from build123d import *

# Parameters (mm, degrees)
F_5_16_CLEARANCE_HOLE1_D = 8.4328
CIRPATTERN1_COUNT        = 8
F_1_2_CLEARANCE_HOLE1_D  = 13.49248
CIRPATTERN2_COUNT        = 2


with BuildPart() as part:
    # Sketch1 → Revolve1 (revolve)
    with BuildSketch(Plane.XY):
        Polygon((-19.431, 0), (-50.8, 0), (-50.8, 12.7), (-19.05, 12.7), (-19.05, 25.4), (0, 25.4), (0, 0), (-15.875, 0), (-15.875, 2.54), (-19.431, 2.54), align=None)
    revolve(axis=Axis((0, 25.4, 0), (0, -1, 0)))

    # Sketch4 → 1/2 NPT Tapped Hole1 (revolve, cut)
    with BuildSketch(Plane(origin=(0, 25.4, 0), x_dir=(0, 0, 1), z_dir=(1, 0, 0))):
        Polygon((0, 0), (0, 25.4), (8.9281, 25.4), (8.9281, 13.462), (9.479726792, 13.462), (9.8827971, 0), align=None)
    revolve(axis=Axis((0, 31.75, 0), (0, -1, 0)), mode=Mode.SUBTRACT)

    # 5/16 Clearance Hole1 (through all)
    with Locations(Plane(origin=(0, 12.7, 0), x_dir=(1, 0, 0), z_dir=(0, 1, 0))):
        with Locations((44.45, 0)):
            f_5_16_clearance_hole1 = Hole(F_5_16_CLEARANCE_HOLE1_D / 2)

    # CirPattern1: 5/16 Clearance Hole1 ×8 about axis
    cirpattern1_axis = Axis((0, 0, 0), (0, 1, 0))
    for i in range(1, CIRPATTERN1_COUNT):
        add(f_5_16_clearance_hole1.rotate(cirpattern1_axis, i * 360 / CIRPATTERN1_COUNT), mode=Mode.SUBTRACT)

    # 1/2 Clearance Hole1 (through all)
    with Locations(Plane(origin=(0, 12.7, 0), x_dir=(1, 0, 0), z_dir=(0, 1, 0))):
        with Locations((-14.580238773, 35.199810189)):
            f_1_2_clearance_hole1 = Hole(F_1_2_CLEARANCE_HOLE1_D / 2)

    # CirPattern2: 1/2 Clearance Hole1 ×2 about axis
    cirpattern2_axis = Axis((0, 0, 0), (0, 1, 0))
    for i in range(1, CIRPATTERN2_COUNT):
        add(f_1_2_clearance_hole1.rotate(cirpattern2_axis, i * 360 / CIRPATTERN2_COUNT), mode=Mode.SUBTRACT)


solid = part.part
Work out the finished part from the listing and answer in its coordinate system (mm). A direction names the side the tool comes from. Round coordinates to 2 decimals unless told otherwise and drop trailing zeros. Write each loop counter-clockwise with the first axis right and the second up, starting at its lowest first coordinate (ties: lowest second). Pieces come first, ordered by that corner, then holes. Notation, with made-up numbers: (52, 7.5) - (71, 7.5) arc R17 ccw to (71, 26.5) - close; hole circle Ø5 at (37.25, 36.5). An arc over 180 degrees is marked (long way). Answer in a Markdown table with one row per item. Add a question column.
1. For faces 1 (the flat face through (6, 11.938, -7)), 2 (the cylindrical face through (29.819, 6.261, -27.535)), 3 (the cylindrical face through (4.21, 1.25, 18.97)), determine the directions among +Z, -Z, +X, -X, +Y, -Y from which every point of the face is accessible in a straight line to the end or side of a thin tool.
2. Given pin 1 (12 mm diameter, centred on x = 28.5, y = 5.5, fed in from -Z); pin 2 (11 mm diameter, centred on x = 44.45, z = 0, fed in from +Y); pin 3 (1.5 mm diameter, centred on y = 6.5, z = -38.5, fed in from -X), each flat-ended and moving along its own axis, determine where each tip first touches the part or whether it passes through.
3. The mould has two halves that part along X. Classify faces 4 (the cylindrical face through (15.12, 19.14, 11.59)), 5 (the cylindrical face through (-0.185, 6.261, -48.662)), 6 (the flat face through (-8, 25.4, 8)): +X half, -X half, draft (parallel to the pull), parting line (faces both ways), or undercut.
4. A cutting plane is placed at A-A, the plane x = 0. Count the separate pieces of the cut face and the enclosed holes in it, and give its area (3 significant figures).
5. A cutting plane is placed at D-D, the plane x = 44.45. Determine the outline of the cut face in (y, z), and give its area (3 significant figures).
6. A cutting plane is placed at C-C, the plane z = -44.45. Determine the outline of the cut face in (x, y), and give its area (3 significant figures).
7. Find the intervals of material crossed by line 1 along X through (y, z) = (1.5, -35); line 2 along X through (y, z) = (13, -1); line 3 along X through (y, z) = (4.75, -1.5), in increasing order. Write a range as from..to.
Worked out:
| question | item | result |
|---|---|---|
| 1 | face 1 | +Y |
| 1 | face 2 | +Y, -Y |
| 1 | face 3 | -Y |
| 2 | pin 1 | z = -45.55 |
| 2 | pin 2 | y = 12.7 |
| 2 | pin 3 | x = -33.99 |
| 3 | face 4 | parting line |
| 3 | face 5 | undercut |
| 3 | face 6 | draft |
| 4 | separate pieces | 4 |
| 4 | enclosed holes | 0 |
| 4 | area | 1,070 mm^2 |
| 5 | outline | (0, -24.59) - (12.7, -24.59) - (12.7, -4.22) - (0, -4.22) - close; (0, 4.22) - (12.7, 4.22) - (12.7, 24.59) - (0, 24.59) - close |
| 5 | area | 518 mm^2 |
| 6 | outline | (-24.59, 0) - (-4.22, 0) - (-4.22, 12.7) - (-24.59, 12.7) - close; (4.22, 0) - (24.59, 0) - (24.59, 12.7) - (4.22, 12.7) - close |
| 6 | area | 518 mm^2 |
| 7 | line 1 | -36.82..-33.68, -29.19..-21.32, -7.84..29.19, 33.68..36.82 |
| 7 | line 2 | -19.02..-9.46, 9.46..19.02 |
| 7 | line 3 | -50.78..-48.39, -40.51..-8.8, 8.8..40.51, 48.39..50.78 |
